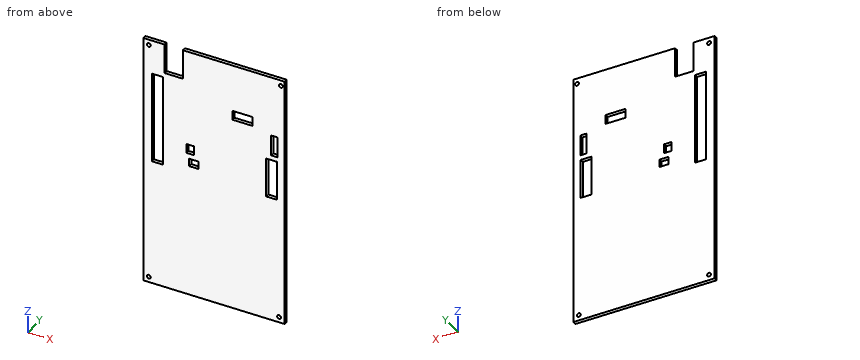
```python
from build123d import *

# Parameters (mm, degrees)
SKETCH_2_R      = 1.05
SKETCH_2_W      = 6
SKETCH_2_H      = 49.2
SKETCH_2_W_2    = 4.15
SKETCH_2_H_2    = 5
SKETCH_2_W_3    = 5
SKETCH_2_H_3    = 4.15
SKETCH_2_W_4    = 11
SKETCH_2_W_5    = 3.5
SKETCH_2_H_4    = 11.2
SKETCH_2_H_5    = 21.3
EXTRUDE_1_DEPTH = 2


with BuildPart() as part:
    # 草图2 → 凸台-拉伸1 (new body)
    with BuildSketch(Plane(origin=(0, 0, 0), x_dir=(1, 0, 0), z_dir=(0, 1, 0))):
        Polygon((77, 0), (0, 0), (0, -136), (11.5, -136), (11.5, -120), (21.5, -120), (21.5, -136), (77, -136), align=None)
        with Locations(Location((3, -133, 0), (0, 0, 270))):
            Circle(SKETCH_2_R, mode=Mode.SUBTRACT)
        with Locations((7.6, -92.9)):
            Rectangle(SKETCH_2_W, SKETCH_2_H, mode=Mode.SUBTRACT)
        with Locations((25.575, -81.5)):
            Rectangle(SKETCH_2_W_2, SKETCH_2_H_2, mode=Mode.SUBTRACT)
        with Locations((27.48, -74.125)):
            Rectangle(SKETCH_2_W_3, SKETCH_2_H_3, mode=Mode.SUBTRACT)
        with Locations((54, -108.1)):
            Rectangle(SKETCH_2_W_4, SKETCH_2_H_2, mode=Mode.SUBTRACT)
        with Locations(Location((75, -133, 0), (0, 0, 270))):
            Circle(SKETCH_2_R, mode=Mode.SUBTRACT)
        with Locations((71.45, -97.9)):
            Rectangle(SKETCH_2_W_5, SKETCH_2_H_4, mode=Mode.SUBTRACT)
        with Locations((70, -79.05)):
            Rectangle(SKETCH_2_W, SKETCH_2_H_5, mode=Mode.SUBTRACT)
        with Locations(Location((3, -3, 0), (0, 0, 270))):
            Circle(SKETCH_2_R, mode=Mode.SUBTRACT)
        with Locations(Location((74, -3, 0), (0, 0, 270))):
            Circle(SKETCH_2_R, mode=Mode.SUBTRACT)
    extrude(amount=EXTRUDE_1_DEPTH)


solid = part.part
```
Source: CAD feature listing. Evaluate the final solid. Frame: model axes, mm. Round coordinates to 2 decimals unless told otherwise and drop trailing zeros. Loops run counter-clockwise (first coordinate to the right, second up) from the corner with the lowest first, then second, coordinate; pieces in that order, holes last. Notation, with made-up numbers: M 18,21.5 L 58,21.5 A19 cw 58,42.5 Z; hole C -34,82.5 d8. An arc over 180 degrees is marked long. Use a Markdown table: item, result. Add a question column.
1. Cut plane C-C, the plane y = 0.9. State how many separate pieces and enclosed holes the cut face has, and give its area (3 significant figures).
2. Cut plane D-D, the plane x = 14. Output: boundary loops of the cut face in (y, z), and give its area (3 significant figures).
3. Cut plane B-B, the plane z = 101. Output: boundary loops of the cut face in (x, y).
4. Cut plane A-A, the plane x = 51.5. Output: boundary loops of the cut face in (y, z).
5. Ray query, line 1 along X through (y, z) = (1.4, 3); line 2 along X through (y, z) = (1.1, 96.5); line 3 along Z through (x, y) = (72.5, 1.55). Return the intervals inside material, ascending. Write a range as [from, to].
Solution:
| question | item | result |
|---|---|---|
| 1 | separate pieces | 1 |
| 1 | enclosed holes | 10 |
| 1 | area | 9,740 mm2 |
| 2 | outline | M 0,0 L 2,0 L 2,120 L 0,120 Z |
| 2 | area | 240 mm2 |
| 3 | outline | M 0,0 L 4.6,0 L 4.6,2 L 0,2 Z; M 10.6,0 L 69.7,0 L 69.7,2 L 10.6,2 Z; M 73.2,0 L 77,0 L 77,2 L 73.2,2 Z |
| 4 | outline | M 0,0 L 2,0 L 2,105.6 L 0,105.6 Z; M 0,110.6 L 2,110.6 L 2,136 L 0,136 Z |
| 5 | line 1 | x = [0, 1.95], [4.05, 72.95], [75.05, 77] |
| 5 | line 2 | x = [0, 4.6], [10.6, 69.7], [73.2, 77] |
| 5 | line 3 | z = [0, 68.4], [89.7, 92.3], [103.5, 136] |
